For this review, use the dimensioned drawing (mm, ordinates from the lowest corner) and the shaded views. A direction names the side the tool comes from. Round coordinates to 2 decimals unless told otherwise and drop trailing zeros. Order: outer loops, then holes, each group sorted by start corner. A loop starts at its lowest first (then second) coordinate and runs counter-clockwise, first axis right, second up. Notation, with made-up numbers: (-22, 3) -> (7, 3) arc R17 cw to (7, 34) -> close; hole circle Ø7 at (-26, 33.5). An arc over 180 degrees is marked (long way). Answer in a Markdown table with one row per item.
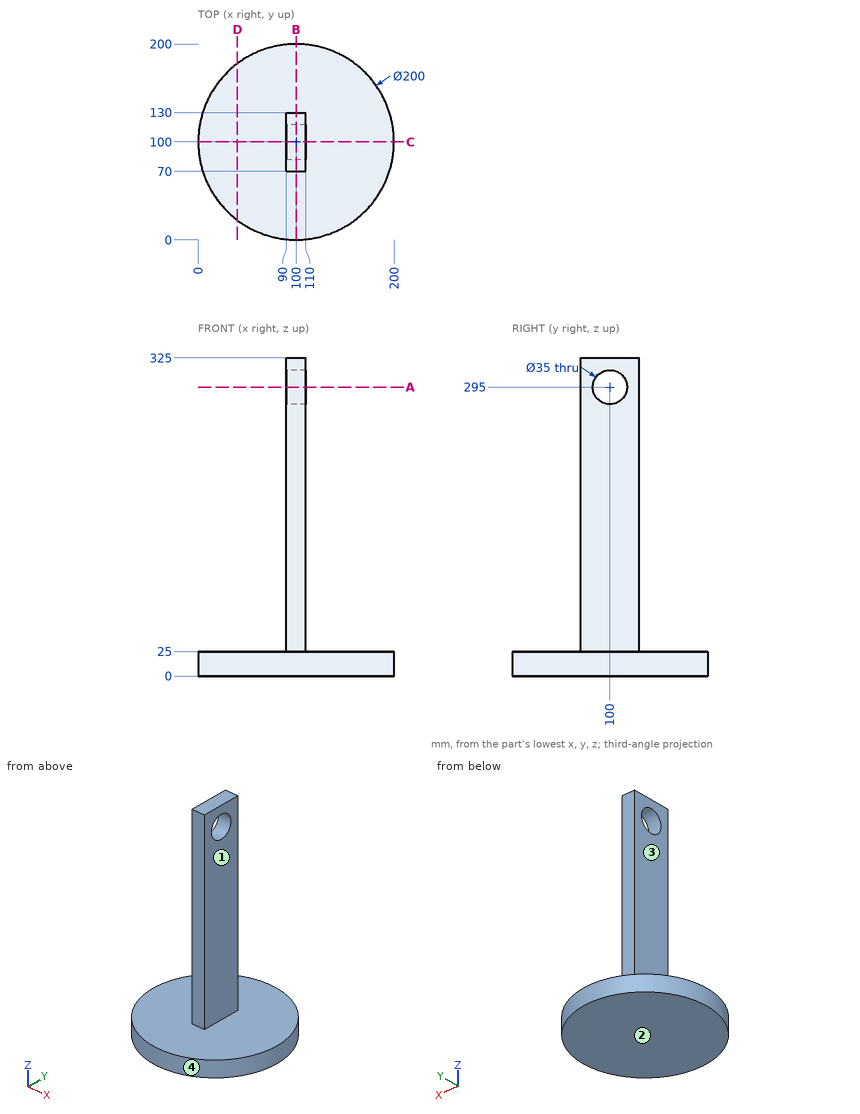
Q1. The part is to be moulded in two halves that separate along Y. For the marked faces 3 and 4, say which applies: +Y half, -Y half, draft (parallel to the pull), parting line (faces both ways), or undercut.
Answer key:
| item | result |
|---|---|
| face 3 | draft |
| face 4 | parting line |
Q2. Take a section at D-D, the plane x = 40. Write out the cut boundary in (y, z).
Answer key:
| item | result |
|---|---|
| outline | (20, 0) -> (180, 0) -> (180, 25) -> (20, 25) -> close |
Q3. Clearance check with flat-ended pins moving along their axes: pin 1 Ø1.5 at (y, z) = (92.5, 268.5) entering from -X; pin 2 Ø6 at (x, z) = (95.5, 104.5) entering from +Y; pin 3 Ø16 at (x, z) = (99.5, 239.5) entering from -Y. State where each tip first meets the part, or that it passes through.
Answer key:
| item | result |
|---|---|
| pin 1 | stops at x = 90 |
| pin 2 | stops at y = 130 |
| pin 3 | stops at y = 70 |
Q4. Take a section at A-A, the plane z = 295. Write out the cut boundary in (x, y), then the cut area to 3 significant figures.
Answer key:
| item | result |
|---|---|
| outline | (90, 70) -> (110, 70) -> (110, 82.5) -> (90, 82.5) -> close; (90, 117.5) -> (110, 117.5) -> (110, 130) -> (90, 130) -> close |
| area | 500 mm^2 |
Q5. To check wall thickness, follow probe 1 along Z at (x, y) = (105, 100); probe 2 along Z at (x, y) = (35, 26.5); probe 3 along X at (y, z) = (120.5, 110). State the ranges of each line that lie inside material, in increasing order.
Answer key:
| item | result |
|---|---|
| probe 1 | z = 0 to 277.5, 312.5 to 325 |
| probe 2 | z = 0 to 25 |
| probe 3 | x = 90 to 110 |
Q6. Take a section at B-B, the plane x = 100. Write out the cut boundary in (y, z), then the cut area to 3 significant figures.
Answer key:
| item | result |
|---|---|
| outline | (0, 0) -> (200, 0) -> (200, 25) -> (130, 25) -> (130, 325) -> (70, 325) -> (70, 25) -> (0, 25) -> close; hole circle Ø35 at (100, 295) |
| area | 22,000 mm^2 |
Q7. Take a section at C-C, the plane y = 100. Write out the cut boundary in (x, z), then the cut area to 3 significant figures.
Answer key:
| item | result |
|---|---|
| outline | (0, 0) -> (200, 0) -> (200, 25) -> (110, 25) -> (110, 277.5) -> (90, 277.5) -> (90, 25) -> (0, 25) -> close; (90, 312.5) -> (110, 312.5) -> (110, 325) -> (90, 325) -> close |
| area | 10,300 mm^2 |
Q8. Tool access review of the marked faces 1 and 2: name each direction out of +Z, -Z, +X, -X, +Y, -Y from which nothing blocks a thin tool from reaching the whole face with its end or side.
Answer key:
| item | result |
|---|---|
| face 1 | +Z, +X, +Y, -Y |
| face 2 | -Z, +X, -X, +Y, -Y |
